from build123d import *

# Parameters (mm, degrees)
SKETCH3_R          = 25.4
CUT_EXTRUDE2_DEPTH = 58.529738397


with BuildPart() as part:
    # Sketch1 → Revolve1 (revolve)
    with BuildSketch(Plane(origin=(0, 0, 0), x_dir=(1, 0, 0), z_dir=(0, 1, 0)), mode=Mode.PRIVATE) as revolve1_sk:
        Polygon((0, 0), (0, 38.1), (-29.21, 38.1), (-29.21, 25.4), (-29.845, 25.4), (-29.845, 12.7), (-30.48, 12.7), (-30.48, 0), align=None)
    revolve(revolve1_sk.sketch.rotate(Axis((0, 0, 0), (0, 0, -1)), 180), axis=Axis((0, 0, 0), (0, 0, -1)))

    # Sketch3 → Cut-Extrude2 (cut, through all)
    with BuildSketch(Plane(origin=(0, 0, -38.1), x_dir=(-1, 0, 0), z_dir=(0, 0, -1))):
        Circle(SKETCH3_R)
    extrude(amount=-CUT_EXTRUDE2_DEPTH, mode=Mode.SUBTRACT)


solid = part.part
Geometry: final body of the model. Coordinates: model frame, mm. A direction names the side the tool comes from. Coordinates: 2 decimals unless noted, no trailing zeros. Write each loop counter-clockwise with the first axis right and the second up, starting at its lowest first coordinate (ties: lowest second). Pieces come first, ordered by that corner, then holes. Notation, with made-up numbers: (86, 62) - (105, 62) arc R26 cw to (105, 99) - close; hole circle Ø1 at (13.5, 36.25). An arc over 180 degrees is marked (long way). Return JSON: item names as keys, results as strings.
Item 1: Section query A-A (y = 0). Output: boundary loops of the cut face in (x, z) (3 decimals), and give its area (3 significant figures).
Completed:
{"outline": "(-30.48, -12.7) - (-29.845, -12.7) - (-29.845, -25.4) - (-29.21, -25.4) - (-29.21, -38.1) - (-25.4, -38.1) - (-25.4, 0) - (-30.48, 0) - close; (25.4, -38.1) - (29.21, -38.1) - (29.21, -25.4) - (29.845, -25.4) - (29.845, -12.7) - (30.48, -12.7) - (30.48, 0) - (25.4, 0) - close", "area": "339 mm2"}
Item 2: Line query: L1, parallel to Y at x = 0, z = -25 (3 decimals); L2, parallel to X at y = -1.5, z = -19; L3, parallel to X at y = 10, z = -4.5. Output: solid intervals per line, ascending.
Completed:
{"L1": "y = -29.845 to -25.4, 25.4 to 29.845", "L2": "x = -29.81 to -25.36, 25.36 to 29.81", "L3": "x = -28.79 to -23.35, 23.35 to 28.79"}
Item 3: Pull-direction query (X, two-part tool) for faces 3 (the face through (5.506, -24.796, -19.317)), 4 (the face through (15.7, -24.63, -31.66)), 5 (the face through (-20.2, 22.4, -12.7)); classes: +X half, -X half, draft (parallel to the pull), parting line (faces both ways), or undercut.
Completed:
{"face 3": "undercut", "face 4": "parting line", "face 5": "draft"}
Item 4: Pin query (flat end, axial travel): pin 1 Ø8 at (y, z) = (5.5, -6) entering from +X; pin 2 Ø8 at (x, z) = (-20.5, -25.5) entering from -Y; pin 3 Ø3 at (y, z) = (16, -15) entering from -X. Return the tip coordinate at first contact, or that it passes through.
Completed:
{"pin 1": "stops at x = 30.44", "pin 2": "stops at y = -24.87", "pin 3": "stops at x = -26.09"}
Item 5: Reachability of faces 1 (the face through (-3.97, -30.22, -6.26)), 2 (the face through (28.47, -8.96, -18.96)) from +Z, -Z, +X, -X, +Y, -Y: full face, straight path, thin tool, end or side. Return the list, or none.
Completed:
{"face 1": "+Z, -Z", "face 2": "-Z"}
